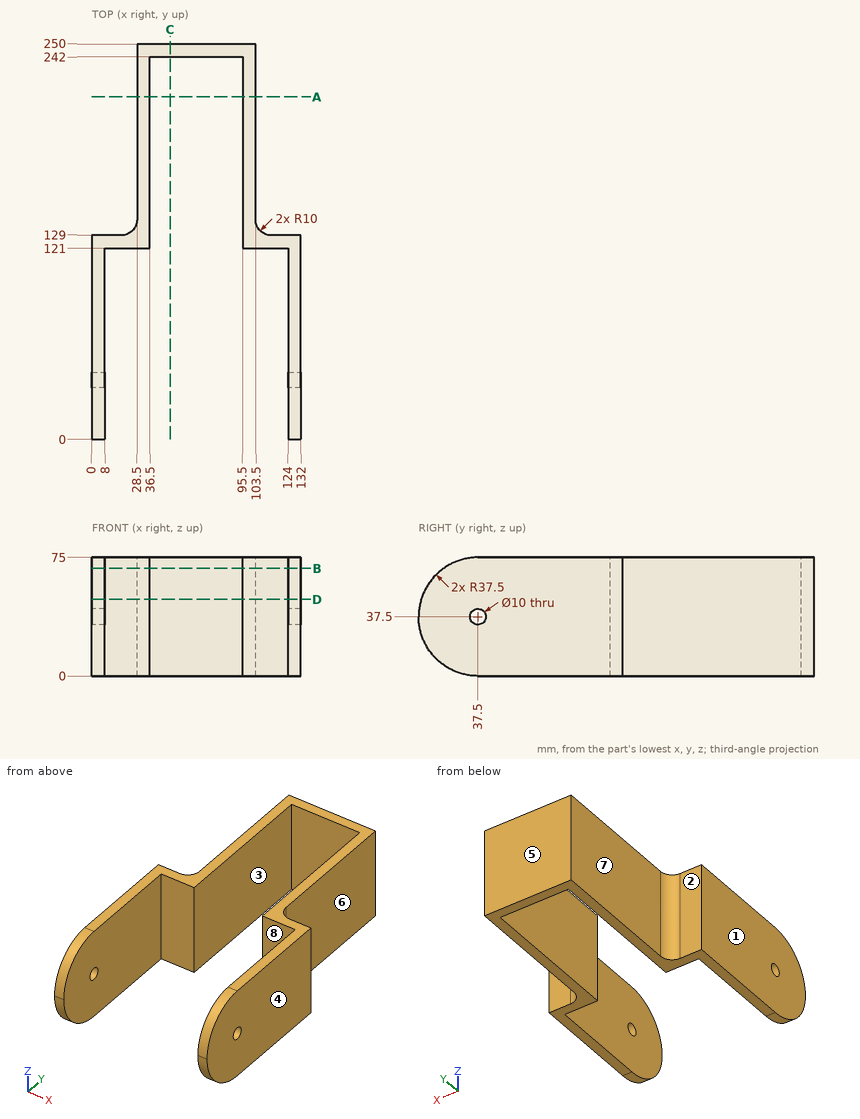
Here's the drawing with two shaded views (mm, measured from the low corner). I have some questions. A direction names the side the tool comes from. Give positions to 0.01 mm unless a question says otherwise; leave off trailing zeros. Order: outer loops, then holes, each group sorted by start corner. A loop starts at its lowest first (then second) coordinate and runs counter-clockwise, first axis right, second up. Notation, with made-up numbers: M -36.5,25.5 L 3.5,25.5 A14 cw 3.5,43.5 Z; hole C 63,48 d2. An arc over 180 degrees is marked long. One line per question, with ' | ' between items.
Item 1: I'm going to push flat-ended pins straight in: pin 1 Ø23 at (x, z) = (108.5, 46.5) entering from -Y; pin 2 Ø2 at (y, z) = (172.5, 22) entering from -X; pin 3 Ø13 at (y, z) = (37.5, 37.5) entering from +X; pin 4 Ø4 at (y, z) = (184, 35.5) entering from +X. Where does each tip first touch, or does it pass through?
Answer block:
pin 1: stops at y = 121 | pin 2: stops at x = 28.5 | pin 3: stops at x = 132 | pin 4: stops at x = 103.5
Item 2: Suppose I cut it at A-A, the plane y = 216.5. Write out the boundary of the cut face in (x, z).
Answer block:
outline: M 28.5,0 L 36.5,0 L 36.5,75 L 28.5,75 Z; M 95.5,0 L 103.5,0 L 103.5,75 L 95.5,75 Z
Item 3: Suppose I cut it at B-B, the plane z = 68. Write out the boundary of the cut face in (x, y).
Answer block:
outline: M 0,15.68 L 8,15.68 L 8,121 L 36.5,121 L 36.5,242 L 95.5,242 L 95.5,121 L 124,121 L 124,15.68 L 132,15.68 L 132,129 L 113.5,129 A10 cw 103.5,139 L 103.5,250 L 28.5,250 L 28.5,139 A10 cw 18.5,129 L 0,129 Z
Item 4: We'd pull the mould along X, two halves only. Please class the marked faces 1, 2 and 3: released by +X, released by -X, zero draft, split by the parting line, or undercut.
Answer block:
face 1: released by -X | face 2: zero draft | face 3: undercut
Item 5: For the marked faces 4, 5, 6, 7 and 8, which set-ups out of +Z, -Z, +X, -X, +Y, -Y let a thin tool reach every point of the face, with its end or its side?
Answer block:
face 4: +Z, -Z, +X, +Y, -Y | face 5: +Z, -Z, +X, -X, +Y | face 6: +Z, -Z, +X, +Y | face 7: +Z, -Z, -X, +Y | face 8: +Z, -Z, -Y
Item 6: Please list where these lines run through material, in increasing order: L1, parallel to X at y = 209.5, z = 50.5; L2, parallel to Y at x = 4, z = 37 (1 decimal); L3, parallel to X at y = 23, z = 60.
Answer block:
L1: x = 28.5 to 36.5, 95.5 to 103.5 | L2: y = 0 to 32.5, 42.5 to 129 | L3: x = 0 to 8, 124 to 132
Item 7: Suppose I cut it at D-D, the plane z = 48.5. Write out the boundary of the cut face in (x, y), then the cut area to 3 significant figures.
Answer block:
outline: M 0,1.65 L 8,1.65 L 8,121 L 36.5,121 L 36.5,242 L 95.5,242 L 95.5,121 L 124,121 L 124,1.65 L 132,1.65 L 132,129 L 113.5,129 A10 cw 103.5,139 L 103.5,250 L 28.5,250 L 28.5,139 A10 cw 18.5,129 L 0,129 Z | area: 4,940 mm2
Item 8: Suppose I cut it at C-C, the plane x = 49.5. Write out the boundary of the cut face in (y, z), then the cut area to 3 significant figures.
Answer block:
outline: M 242,0 L 250,0 L 250,75 L 242,75 Z | area: 600 mm2
